Verification items for the finished model (mm, model axes). Face numbers are marked on the shaded views. A direction names the side the tool comes from. Give positions to 0.01 mm unless a question says otherwise; leave off trailing zeros. Loops run counter-clockwise (first coordinate to the right, second up) from the corner with the lowest first, then second, coordinate; pieces in that order, holes last. Notation, with made-up numbers: (-14, -31.75) - (21, -31.75) arc R5 cw to (21, -25.75) - close; hole circle Ø10 at (43, -30). An arc over 180 degrees is marked (long way). One line per item, written item: value. Start each with the question number.
1. Mould release check, pull along X, two halves, no side actions. Record for the marked faces 1, 2 and 3: pulls with the +X half, pulls with the -X half, needs draft (parallel to the pull), parting line crosses it, or undercut.
2. Sectioned sample at B-B (z = 10.5). Record the cut outline in (x, y) (3 decimals).
3. Access from +Z, -Z, +X, -X, +Y, -Y to the whole of each face (thin tool, end or side, straight path). Record for the marked faces 4, 5 and 6.
4. Sectioned sample at C-C (y = 2.5). Count the separate pieces of the cut face and the enclosed holes in it, plus the area to 3 significant figures.
5. Gauge pin test, flat ends, axial feed: pin 1 (8 mm diameter, centred on x = 0.5, z = -3, fed in from +Y); pin 2 (0.8 mm diameter, centred on x = -5, y = -1.5, fed in from +Z); pin 3 (1 mm diameter, centred on x = -10, z = 1, fed in from -Y) (3 decimals). Record the tip position at first contact, or that the pin passes through.
6. Scan lines: L1, parallel to X at y = 1.3, z = 0 (3 decimals); L2, parallel to X at y = 6.75, z = 0 (3 decimals); L3, parallel to X at y = 9.75, z = 4.75 (3 decimals). Record each from-to range of solid material in increasing order. Write a range as [from, to].
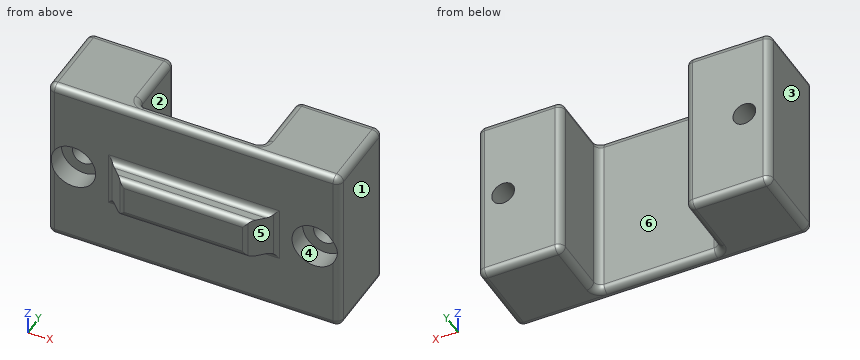
from build123d import *

# Parameters (mm, degrees)
SKETCH_1_W           = 42.43
SKETCH_1_H           = 25
EXTRUDE_1_DEPTH      = 2
SKETCH_2_W           = 12.22
SKETCH_2_H           = 25
EXTRUDE_2_DEPTH      = 10
SKETCH_3_R           = 1.65
CUT_EXTRUDE_1_DEPTH  = 28.392083254
EXTRUDE_3_DEPTH      = 3
EXTRUDE_3_DEPTH_BACK = 3
FILLET_2_R           = 1
SKETCH_5_R           = 3.25
CUT_EXTRUDE_2_DEPTH  = 3


with BuildPart() as part:
    # ｽｹｯﾁ1 → ﾎﾞｽ - 押し出し1 (new body)
    with BuildSketch(Plane(origin=(0, 0, 0), x_dir=(1, 0, 0), z_dir=(0, 1, 0))):
        Rectangle(SKETCH_1_W, SKETCH_1_H)
    extrude(amount=EXTRUDE_1_DEPTH)

    # ｽｹｯﾁ2 → ﾎﾞｽ - 押し出し2 (add)
    with BuildSketch(Plane(origin=(0, 2, 0), x_dir=(1, 0, 0), z_dir=(0, 1, 0))):
        with Locations((-15.105, 0)):
            Rectangle(SKETCH_2_W, SKETCH_2_H)
        with Locations((15.105, 0)):
            Rectangle(SKETCH_2_W, SKETCH_2_H)
    extrude(amount=EXTRUDE_2_DEPTH)

    # ｽｹｯﾁ3 → ｶｯﾄ - 押し出し1 (cut, through all)
    with BuildSketch(Plane(origin=(0, 12, 0), x_dir=(1, 0, 0), z_dir=(0, 1, 0))):
        with Locations(Location((-17.495, 0, 0), (0, 0, 270))):
            Circle(SKETCH_3_R)
        with Locations(Location((17.505, 0, 0), (0, 0, 270))):
            Circle(SKETCH_3_R)
    extrude(amount=-CUT_EXTRUDE_1_DEPTH, mode=Mode.SUBTRACT)

    # ｽｹｯﾁ4 → ﾎﾞｽ - 押し出し3 (add, two sides: drawn at the far end of the back side and taken through both)
    with BuildSketch(Plane.XY.offset(-EXTRUDE_3_DEPTH_BACK)):
        Polygon((-11.995, 0), (-8.995, -3), (8.995, -3), (11.995, 0), align=None)
    extrude(amount=EXTRUDE_3_DEPTH + EXTRUDE_3_DEPTH_BACK)

    # ﾌｨﾚｯﾄ2
    fillet_2_edges = [part.edges().sort_by_distance(p)[0] for p in [
        (0, 2, 12.5),
        (-8.995, 2, 0),
        (-8.995, 7, 12.5),
        (-8.995, 7, -12.5),
        (-21.215, 12, 0),
        (-15.105, 12, 12.5),
        (-8.995, 12, 0),
        (-15.105, 12, -12.5),
        (0, 2, -12.5),
        (8.995, 2, 0),
        (8.995, 7, -12.5),
        (8.995, 7, 12.5),
        (21.215, 12, 0),
        (15.105, 12, -12.5),
        (8.995, 12, 0),
        (15.105, 12, 12.5),
        (-8.995, -3, 0),
        (-11.995, 0, 0),
        (0, 0, 3),
        (11.995, 0, 0),
        (0, 0, 12.5),
        (8.995, -3, 0),
        (0, -3, -3),
        (0, 0, -3),
        (0, -3, 3),
        (-21.215, 0, 0),
        (0, 0, -12.5),
        (21.215, 0, 0),
        (21.215, 6, 12.5),
        (-21.215, 6, 12.5),
        (-21.215, 6, -12.5),
        (21.215, 6, -12.5),
    ]]
    fillet(fillet_2_edges, radius=FILLET_2_R - 0.0001)  # a hair under: the kernel refuses the full size

    # ｽｹｯﾁ5 → ｶｯﾄ - 押し出し2 (cut)
    with BuildSketch(Plane(origin=(0, 0, 0), x_dir=(-1, 0, 0), z_dir=(0, -1, 0))):
        with Locations(Location((-17.505, 0, 0), (0, 0, 90))):
            Circle(SKETCH_5_R)
        with Locations(Location((17.495, 0, 0), (0, 0, 90))):
            Circle(SKETCH_5_R)
    extrude(amount=-CUT_EXTRUDE_2_DEPTH, mode=Mode.SUBTRACT)


solid = part.part
Results are:
1. face 1: pulls with the +X half
1. face 2: undercut
1. face 3: pulls with the -X half
2. outline: (-21.215, 1) arc R1 ccw to (-20.215, 0) - (20.215, 0) arc R1 ccw to (21.215, 1) - (21.215, 11) arc R1 ccw to (20.215, 12) - (9.995, 12) arc R1 ccw to (8.995, 11) - (8.995, 3) arc R1 cw to (7.995, 2) - (-7.995, 2) arc R1 cw to (-8.995, 3) - (-8.995, 11) arc R1 ccw to (-9.995, 12) - (-20.215, 12) arc R1 ccw to (-21.215, 11) - close
3. face 4: -Y
3. face 5: +Z, -Z, +X, -Y
3. face 6: +Z, -Z, +Y
4. separate pieces: 2
4. enclosed holes: 2
4. area: 550 mm^2
5. pin 1: stops at y = 2
5. pin 2: stops at z = 3
5. pin 3: stops at y = -2.495
6. L1: x = [-21.215, -20.745], [-14.245, 14.255], [20.755, 21.215]
6. L2: x = [-21.215, -19.145], [-15.845, -8.995], [8.995, 15.855], [19.155, 21.215]
6. L3: x = [-21.215, -8.995], [8.995, 21.215]
